Source: three-view drawing plus pictorial views. Frame: mm from the lowest corner of the part. Give positions to 0.01 mm unless a question says otherwise; leave off trailing zeros. Loops run counter-clockwise (first coordinate to the right, second up) from the corner with the lowest first, then second, coordinate; pieces in that order, holes last. Notation, with made-up numbers: (4.25, -3.5) - (29.25, -3.5) arc R33 ccw to (29.25, 31.5) - close; hole circle Ø7 at (88, 42.5). An arc over 180 degrees is marked (long way). Write each question's results on one line, items separated by ' | '. Start each with the question number.
(1) Material intervals for line 1 along X through (y, z) = (54, 5); line 2 along Y through (x, z) = (1642, 60.5), sorted ascending. Write a range as [from, to].
(2) Cut plane C-C on x = 1463. Return the cut outline in (y, z).
(3) Contact query for flat-ended pins moving along their axis: pin 1 (6 mm diameter, centred on x = 301.5, z = 30, fed in from -Y); pin 2 (10 mm diameter, centred on x = 1664.5, z = 76, fed in from +Y); pin 3 (4 mm diameter, centred on x = 716.5, y = 73, fed in from -Z). Output: stop coordinate, or through.
(4) Cut plane A-A on z = 72. Return the cut outline in (x, y), then the cut area to 3 significant figures.
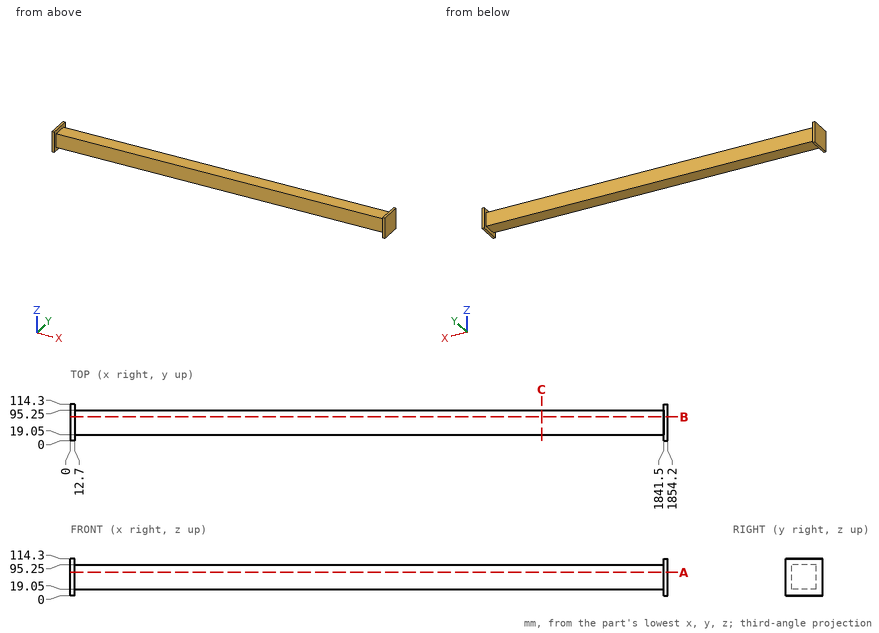
Ans:
1) line 1: [0, 12.7], [1841.5, 1854.2] | line 2: [19.05, 95.25]
2) outline: (19.05, 19.05) - (95.25, 19.05) - (95.25, 95.25) - (19.05, 95.25) - close
3) pin 1: y = 19.05 | pin 2: y = 95.25 | pin 3: z = 19.05
4) outline: (0, 0) - (12.7, 0) - (12.7, 19.05) - (1841.5, 19.05) - (1841.5, 0) - (1854.2, 0) - (1854.2, 114.3) - (1841.5, 114.3) - (1841.5, 95.25) - (12.7, 95.25) - (12.7, 114.3) - (0, 114.3) - close | area: 142,000 mm^2
